Model file for the job. Use its own axes, mm. Give positions to 0.01 mm unless a question says otherwise; leave off trailing zeros. Write each loop counter-clockwise with the first axis right and the second up, starting at its lowest first coordinate (ties: lowest second). Pieces come first, ordered by that corner, then holes. Notation, with made-up numbers: (70.5, 64) - (77.5, 64) arc R10 cw to (77.5, 79) - close; hole circle Ø10 at (85, -16). An arc over 180 degrees is marked (long way). One line per item, written item: value. Start each with the question number.
(1) Cut at A-A, the plane x = 19.5. List the corners of the cut face in (y, z), and give its area (3 significant figures).
(2) Probe L1, parallel to X at y = -2.5, z = 7.75; L2, parallel to Y at x = 35, z = 4.25; L3, parallel to Y at x = 1.5, z = 2. List the from-to ranges inside material, lowest first.
(3) Drop a flat-ended pin along its axis: P1, Ø8, axis at x = 0, y = -14, coming from the -Z side. Give the stop position or say it passes through.
(4) Cut at B-B, the plane z = 8.75. List the corners of the cut face in (x, y).
(5) Cut at C-C, the plane x = -6. List the corners of the cut face in (y, z), and give its area (3 significant figures).
from build123d import *

# Parameters (mm, degrees)
F0_W     = 60
F0_H     = 20
F0_R     = 1.75
F0_R_2   = 1.8
F0_R_3   = 1.85
F0_R_4   = 1.9
F0_R_5   = 1.95
F0_R_6   = 2
F0_W_2   = 2.181272
F0_H_2   = 2.106054
F1_DEPTH = 10


with BuildPart() as f1:
    # F0 (on Top) → F1 (new body)
    with BuildSketch(Plane.XY):
        with Locations((15.278291, -10.103558)):
            Rectangle(F0_W, F0_H)
        with Locations((-6.221709, -10.103558)):
            Circle(F0_R, mode=Mode.SUBTRACT)
        with Locations((2.278291, -10.103558)):
            Circle(F0_R_2, mode=Mode.SUBTRACT)
        with Locations((10.778291, -10.103558)):
            Circle(F0_R_3, mode=Mode.SUBTRACT)
        with Locations((19.278291, -10.103558)):
            Circle(F0_R_4, mode=Mode.SUBTRACT)
        with Locations((27.778291, -10.103558)):
            Circle(F0_R_5, mode=Mode.SUBTRACT)
        with Locations((36.278291, -10.103558)):
            Circle(F0_R_6, mode=Mode.SUBTRACT)
        with Locations((-12.932548, -1.785417)):
            Rectangle(F0_W_2, F0_H_2, mode=Mode.SUBTRACT)
    extrude(amount=F1_DEPTH)


solid = f1.part
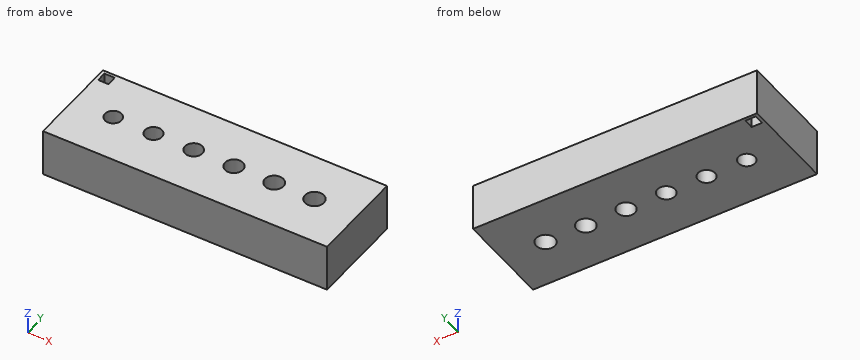
Answers follow:
1. outline: (-20.1, 0) - (-11.99, 0) - (-11.99, 10) - (-20.1, 10) - close; (-8.22, 0) - (-0.1, 0) - (-0.1, 10) - (-8.22, 10) - close
1. area: 162 mm²
2. L1: x = -14.72 to -14.02, -11.84 to 45.28
2. L2: y = -20.1 to -11.64, -8.57 to -0.1
2. L3: y = -20.1 to -11.73, -8.48 to -0.1
3. P1: stops at z = 0
4. outline: (-14.72, -20.1) - (45.28, -20.1) - (45.28, -0.1) - (-14.72, -0.1) - close; hole (-14.02, -2.84) - (-11.84, -2.84) - (-11.84, -0.73) - (-14.02, -0.73) - close; hole circle Ø3.5 at (-6.22, -10.1); hole circle Ø3.6 at (2.28, -10.1); hole circle Ø3.7 at (10.78, -10.1); hole circle Ø3.8 at (19.28, -10.1); hole circle Ø3.9 at (27.78, -10.1); hole circle Ø4 at (36.28, -10.1)
5. outline: (-20.1, 0) - (-11.84, 0) - (-11.84, 10) - (-20.1, 10) - close; (-8.37, 0) - (-0.1, 0) - (-0.1, 10) - (-8.37, 10) - close
5. area: 165 mm²
